Could you check a few things on this model? Use its own coordinates, in mm. A direction names the side the tool comes from. Coordinates: 2 decimals unless noted, no trailing zeros. Order: outer loops, then holes, each group sorted by start corner. A loop starts at its lowest first (then second) coordinate and runs counter-clockwise, first axis right, second up. Notation, with made-up numbers: (61, 71.5) -> (67, 71.5) arc R21 ccw to (67, 78.5) -> close; hole circle Ø2 at (-35.5, 19.25). An arc over 180 degrees is marked (long way). Return JSON: item names as keys, results as strings. Group by question number.
from build123d import *

# Parameters (mm, degrees)
EXTRUDE_1_DEPTH     = 6
SKETCH_2_W          = 10
SKETCH_2_H          = 2
EXTRUDE_2_DEPTH     = 10
SKETCH_3_W          = 10
SKETCH_3_H          = 2
EXTRUDE_3_DEPTH     = 10
SKETCH_4_R          = 2.040020597
SKETCH_4_R_2        = 2
CUT_EXTRUDE_1_DEPTH = 9
CUT_EXTRUDE_START   = -9
SKETCH_5_R          = 2
CUT_EXTRUDE_2_DEPTH = 9
SKETCH_7_R          = 2.206948318
SKETCH_7_R_2        = 2
SKETCH_7_R_3        = 2.004801963
CUT_EXTRUDE_3_DEPTH = 9


with BuildPart() as part:
    # 草图1 → 凸台-拉伸1 (new body)
    with BuildSketch(Plane.XY):
        Polygon((-405.306796117, 348.186737633), (-520.906796117, 348.186737633), (-520.906796117, 264.386737633), (-405.306796117, 264.386737633), (-405.306796117, 274.386737633), (-498.306796117, 274.386737633), (-498.306796117, 334.386737633), (-405.306796117, 334.386737633), align=None)
    extrude(amount=-EXTRUDE_1_DEPTH)

    # 草图2 → 凸台-拉伸2 (add)
    with BuildSketch(Plane(origin=(0, 0, -6), x_dir=(-1, 0, 0), z_dir=(0, 0, -1))):
        with Locations((505.906796117, 347.186737633)):
            Rectangle(SKETCH_2_W, SKETCH_2_H)
        with Locations((505.906796117, 265.386737633)):
            Rectangle(SKETCH_2_W, SKETCH_2_H)
    extrude(amount=EXTRUDE_2_DEPTH)

    # 草图3 → 凸台-拉伸3 (add)
    with BuildSketch(Plane(origin=(0, 0, -6), x_dir=(-1, 0, 0), z_dir=(0, 0, -1))):
        with Locations((425.306796117, 347.186737633)):
            Rectangle(SKETCH_3_W, SKETCH_3_H)
        with Locations((425.306796117, 265.386737633)):
            Rectangle(SKETCH_3_W, SKETCH_3_H)
    extrude(amount=EXTRUDE_3_DEPTH)

    # 草图4 → 切除-拉伸1 (cut)
    with BuildSketch(Plane(origin=(0, 348.186737633, 0), x_dir=(1, 0, 0), z_dir=(0, 1, 0))):
        with Locations(Location((-425.380170541, 11, 0), (0, 0, 270))):
            Circle(SKETCH_4_R)
        with Locations(Location((-505.95276467, 11, 0), (0, 0, 270))):
            Circle(SKETCH_4_R_2)
    extrude(amount=-CUT_EXTRUDE_1_DEPTH, mode=Mode.SUBTRACT)

    # 草图5 → 切除-拉伸2 (cut)
    with BuildSketch(Plane.XZ.offset(-264.386737633).offset(CUT_EXTRUDE_START)):
        with Locations(Location((-505.95276467, -11, 0), (0, 0, 90))):
            Circle(SKETCH_5_R)
        with Locations(Location((-425.380170541, -11, 0), (0, 0, 270))):
            Circle(SKETCH_5_R)
    extrude(amount=CUT_EXTRUDE_2_DEPTH, mode=Mode.SUBTRACT)

    # 草图7 → 切除-拉伸3 (cut)
    with BuildSketch(Plane.XY):
        with Locations((-494.306796117, 339.386737633)):
            Circle(SKETCH_7_R)
        with Locations((-409.306796117, 339.386737633)):
            Circle(SKETCH_7_R_2)
        with Locations((-409.306796117, 269.386737633)):
            Circle(SKETCH_7_R_3)
        with Locations((-494.306796117, 269.386737633)):
            Circle(SKETCH_7_R_2)
    extrude(amount=-CUT_EXTRUDE_3_DEPTH, mode=Mode.SUBTRACT)


solid = part.part
Q1. I want a section at C-C on y = 306.5. Please give me the cut outline in (x, z).
Q2. I want a section at A-A on x = -460.5. Please give me the cut outline in (y, z), and give its area (3 significant figures).
Q3. On a 3-axis mill with a long thin cutter (end or side, diameter ignored), from which of +Z, -Z, +X, -X, +Y, -Y can I reach the whole of each face in a straight line? I mean faces 1 (the flat face through (-462, 348.187, -4)), 2 (the flat face through (-423, 266.387, -11)), 3 (the flat face through (-452, 334.387, -3)). Say none if no direction works.
Q4. I want a section at B-B on z = -14.25. Please give me the cut outline in (x, y).
Q5. We'd pull the mould along Y, two halves only. Please class faces 4 (the flat face through (-505.8, 266.387, -13.2)), 5 (the flat face through (-464, 264.387, -4)), 6 (the cylindrical face through (-427.372, 347.201, -11.442)): pulls with the +Y half, pulls with the -Y half, needs draft (parallel to the pull), parting line crosses it, or undercut.
Q6. I need wall thicknesses on line 1 along Y through (x, z) = (-421, -10.5); line 2 along Y through (x, z) = (-420, -4); line 3 along X through (y, z) = (302, -3.75). Which ranges of each line are inside material? Lowest first, please. Write a range as from..to.
Q7. I'm going to push flat-ended pins straight in: pin 1 Ø5.5 at (x, z) = (-425.38, -11) entering from -Y; pin 2 Ø1 at (y, z) = (347, -12) entering from -X; pin 3 Ø1.6 at (y, z) = (347, -12) entering from +X; pin 4 Ø10 at (x, y) = (-443.5, 282) entering from +Z. Where does each tip first touch, or does it pass through?
Response values:
{
 "1": {"outline": "(-520.91, -6) -> (-498.31, -6) -> (-498.31, 0) -> (-520.91, 0) -> close"},
 "2": {"outline": "(264.39, -6) -> (274.39, -6) -> (274.39, 0) -> (264.39, 0) -> close; (334.39, -6) -> (348.19, -6) -> (348.19, 0) -> (334.39, 0) -> close", "area": "143 mm²"},
 "3": {"face 1": "+Z, -Z, +X, -X, +Y", "face 2": "-Z, +X, -X", "face 3": "+Z, -Z, +X"},
 "4": {"outline": "(-510.91, 264.39) -> (-500.91, 264.39) -> (-500.91, 266.39) -> (-510.91, 266.39) -> close; (-510.91, 346.19) -> (-500.91, 346.19) -> (-500.91, 348.19) -> (-510.91, 348.19) -> close; (-430.31, 264.39) -> (-420.31, 264.39) -> (-420.31, 266.39) -> (-430.31, 266.39) -> close; (-430.31, 346.19) -> (-420.31, 346.19) -> (-420.31, 348.19) -> (-430.31, 348.19) -> close"},
 "5": {"face 4": "undercut", "face 5": "pulls with the -Y half", "face 6": "needs draft"},
 "6": {"line 1": "y = 264.39..266.39, 346.19..348.19", "line 2": "y = 264.39..274.39, 334.39..348.19", "line 3": "x = -520.91..-498.31"},
 "7": {"pin 1": "stops at y = 264.39", "pin 2": "stops at x = -510.91", "pin 3": "stops at x = -420.31", "pin 4": "passes through"}
}
